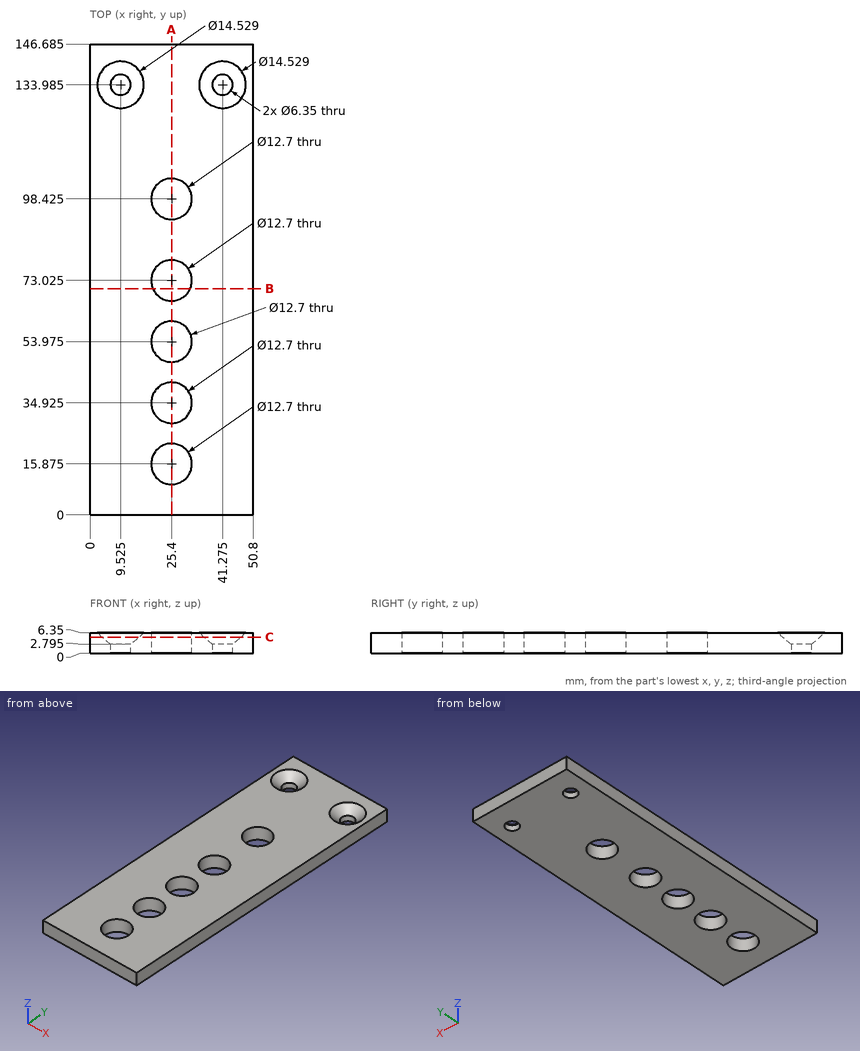
Geometry check sheet. Reference: drawing and pictorial views, mm from the part's lowest x, y, z. Coordinates: 2 decimals unless noted, no trailing zeros. Write each loop counter-clockwise with the first axis right and the second up, starting at its lowest first coordinate (ties: lowest second). Pieces come first, ordered by that corner, then holes. Notation, with made-up numbers: (61, 23.5) -> (93, 23.5) arc R11 cw to (93, 34.5) -> close; hole circle Ø1 at (31, 32.25). An arc over 180 degrees is marked (long way). Use a Markdown table: item, result.
1. Go/stop test with a flat-tipped pin: pin 1 Ø8.5 at (x, y) = (41.275, 133.985) entering from +Z. Record where the tip stops, or that it passes through.
Reported:
| item | result |
|---|---|
| pin 1 | stops at z = 3.73 |
2. Sectioned sample at B-B (y = 70.5). Enter the section's corners in (x, z).
Reported:
| item | result |
|---|---|
| outline | (0, 0) -> (19.57, 0) -> (19.57, 6.35) -> (0, 6.35) -> close; (31.23, 0) -> (50.8, 0) -> (50.8, 6.35) -> (31.23, 6.35) -> close |
3. Scan lines: line 1 along Y through (x, z) = (25.4, 3.75) (3 decimals); line 2 along X through (y, z) = (137, 4.5); line 3 along X through (y, z) = (72.5, 4). Record each from-to range of solid material in increasing order.
Reported:
| item | result |
|---|---|
| line 1 | y = 0 to 9.525, 22.225 to 28.575, 41.275 to 47.625, 60.325 to 66.675, 79.375 to 92.075, 104.775 to 146.685 |
| line 2 | x = 0 to 5.37, 13.68 to 37.12, 45.43 to 50.8 |
| line 3 | x = 0 to 19.07, 31.73 to 50.8 |
4. Sectioned sample at C-C (z = 5). Give the number of separate pieces and of enclosed holes in the cut face, plus the area to 3 significant figures.
Reported:
| item | result |
|---|---|
| separate pieces | 1 |
| enclosed holes | 7 |
| area | 6,610 mm2 |
5. Sectioned sample at A-A (x = 25.4). Enter the section's corners in (y, z) (3 decimals), plus the area to 3 significant figures.
Reported:
| item | result |
|---|---|
| outline | (0, 0) -> (9.525, 0) -> (9.525, 6.35) -> (0, 6.35) -> close; (22.225, 0) -> (28.575, 0) -> (28.575, 6.35) -> (22.225, 6.35) -> close; (41.275, 0) -> (47.625, 0) -> (47.625, 6.35) -> (41.275, 6.35) -> close; (60.325, 0) -> (66.675, 0) -> (66.675, 6.35) -> (60.325, 6.35) -> close; (79.375, 0) -> (92.075, 0) -> (92.075, 6.35) -> (79.375, 6.35) -> close; (104.775, 0) -> (146.685, 0) -> (146.685, 6.35) -> (104.775, 6.35) -> close |
| area | 528 mm2 |
